Source: CAD feature listing. Evaluate the final solid. Frame: model axes, mm. Coordinates: 2 decimals unless noted, no trailing zeros. Order: outer loops, then holes, each group sorted by start corner. A loop starts at its lowest first (then second) coordinate and runs counter-clockwise, first axis right, second up. Notation, with made-up numbers: (31.5, -6) - (86.5, -6) arc R25 cw to (86.5, 20) - close; hole circle Ø1 at (45.5, -2.5). An arc over 180 degrees is marked (long way). One line per question, with ' | ' between items.
from build123d import *

# Parameters (mm, degrees)
F0_R     = 1.5
F1_DEPTH = 5
F2_DEPTH = 5
F3_R     = 22
F4_DEPTH = 6


with BuildPart() as f1:
    # F0 (on Top) → F1 (new body)
    with BuildSketch(Plane.XY):
        with BuildLine():
            ThreePointArc((-26.6379310345, -4.4068844099), (-27, 0), (-26.6379310345, 4.4068844099))
            ThreePointArc((-26.6379310345, 4.4068844099), (-34, 0), (-26.6379310345, -4.4068844099))
        make_face()
        with Locations((-29, 0)):
            Circle(F0_R, mode=Mode.SUBTRACT)
    extrude(amount=F1_DEPTH)



with BuildPart() as f1b:
    # F0 (on Top) → F1, piece 2 (new body)
    with BuildSketch(Plane.XY):
        with BuildLine():
            ThreePointArc((26.6379310345, 4.4068844099), (26.9093305187, 2.21086658), (27, 0))
            ThreePointArc((27, 0), (26.9093305187, -2.21086658), (26.6379310345, -4.4068844099))
            ThreePointArc((26.6379310345, -4.4068844099), (31.5680396388, -4.2901249881), (34, 0))
            ThreePointArc((34, 0), (31.5680396388, 4.2901249881), (26.6379310345, 4.4068844099))
        make_face()
        with Locations((29, 0)):
            Circle(F0_R, mode=Mode.SUBTRACT)
    extrude(amount=F1_DEPTH)


with BuildPart() as f1_1:
    add(f1.part)

    add(f1b.part)  # F2 merges F1b
    # F0 (on Top) → F2 (join)
    with BuildSketch(Plane.XY):
        with BuildLine():
            ThreePointArc((-24, 0), (-24.7098750119, 2.5680396388), (-26.6379310345, 4.4068844099))
            ThreePointArc((-26.6379310345, 4.4068844099), (-27, 0), (-26.6379310345, -4.4068844099))
            ThreePointArc((-26.6379310345, -4.4068844099), (-24.7098750119, -2.5680396388), (-24, 0))
        make_face()
        with BuildLine():
            ThreePointArc((26.6379310345, -4.4068844099), (26.9093305187, -2.21086658), (27, 0))
            ThreePointArc((27, 0), (26.9093305187, 2.21086658), (26.6379310345, 4.4068844099))
            ThreePointArc((26.6379310345, 4.4068844099), (24, 0), (26.6379310345, -4.4068844099))
        make_face()
        with BuildLine():
            ThreePointArc((26.6379310345, -4.4068844099), (24, 0), (26.6379310345, 4.4068844099))
            ThreePointArc((26.6379310345, 4.4068844099), (0, 27), (-26.6379310345, 4.4068844099))
            ThreePointArc((-26.6379310345, 4.4068844099), (-24.7098750119, 2.5680396388), (-24, 0))
            ThreePointArc((-24, 0), (-24.7098750119, -2.5680396388), (-26.6379310345, -4.4068844099))
            ThreePointArc((-26.6379310345, -4.4068844099), (0, -27), (26.6379310345, -4.4068844099))
        make_face()
    extrude(amount=F2_DEPTH)

    # F3 (on face) → F4 (cut)
    with BuildSketch(Plane.XY.offset(5)):
        Circle(F3_R)
    extrude(amount=-F4_DEPTH, mode=Mode.SUBTRACT)


solid = f1_1.part
(1) Material intervals for L1, parallel to Y at x = -29, z = 1.4; L2, parallel to Y at x = -11, z = 4.35; L3, parallel to X at y = -8.5, z = 3.6, sorted ascending. Write a range as from..to.
Taken from the geometry:
L1: y = -5..-1.5, 1.5..5 | L2: y = -24.66..-19.05, 19.05..24.66 | L3: x = -25.63..-20.29, 20.29..25.63
(2) Cut plane C-C (y = 19). Return the cut outline in (x, z).
Taken from the geometry:
outline: (-19.18, 0) - (-11.09, 0) - (-11.09, 5) - (-19.18, 5) - close; (11.09, 0) - (19.18, 0) - (19.18, 5) - (11.09, 5) - close
(3) Cut plane B-B (z = 2.8). Return the cut outline in (x, y).
Taken from the geometry:
outline: (-26.64, -4.41) arc R27 ccw to (26.64, -4.41) arc R5 ccw (long way) to (26.64, 4.41) arc R27 ccw to (-26.64, 4.41) arc R5 ccw (long way) to start; hole circle Ø3 at (-29, 0); hole circle Ø44 at (0, 0); hole circle Ø3 at (29, 0)
(4) Pull-direction query (Y, two-part tool) for faces 1 (the cylindrical face through (-4.769, -21.477, 2.535)), 2 (the flat face through (2.4, 22.1, 0)), 3 (the cylindrical face through (-0.532, -26.995, 2.465)); classes: pulls with the +Y half, pulls with the -Y half, needs draft (parallel to the pull), parting line crosses it, or undercut.
Taken from the geometry:
face 1: undercut | face 2: needs draft | face 3: pulls with the -Y half
(5) Pin query (flat end, axial travel): P1, Ø4, axis at x = -14, y = -16, coming from the -Z side; P2, Ø2.5, axis at x = -29, y = 0, coming from the -Z side. Return the tip coordinate at first contact, or that it passes through.
Taken from the geometry:
P1: stops at z = 0 | P2: passes through
(6) Cut plane A-A (x = 0). Return the cut outline in (y, z), and give its area (3 significant figures).
Taken from the geometry:
outline: (-27, 0) - (-22, 0) - (-22, 5) - (-27, 5) - close; (22, 0) - (27, 0) - (27, 5) - (22, 5) - close | area: 50.0 mm²
(7) Cut plane D-D (y = -23). Return the cut outline in (x, z), and give its area (3 significant figures).
Taken from the geometry:
outline: (-14.14, 0) - (14.14, 0) - (14.14, 5) - (-14.14, 5) - close | area: 141 mm²
